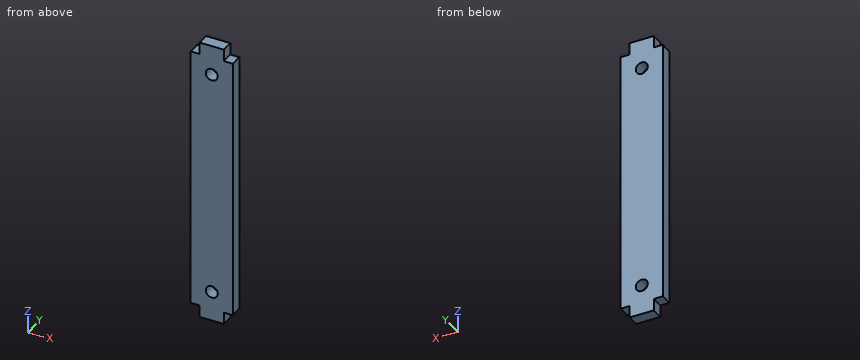
```python
from build123d import *

# Parameters (mm, degrees)
SKETCH1_W           = 17.78
SKETCH1_H           = 111.76
SKETCH1_R           = 2.54
SKETCH1_W_2         = 10.16
SKETCH1_H_2         = 5.08
BOSS_EXTRUDE1_DEPTH = 5.08


with BuildPart() as part:
    # Sketch1 → Boss-Extrude1 (new body)
    with BuildSketch(Plane(origin=(0, 0, 0), x_dir=(1, 0, 0), z_dir=(0, 1, 0))):
        Rectangle(SKETCH1_W, SKETCH1_H)
        with Locations((0, 48.26)):
            Circle(SKETCH1_R, mode=Mode.SUBTRACT)
        with Locations((0, -48.26)):
            Circle(SKETCH1_R, mode=Mode.SUBTRACT)
        with Locations((0, 58.42)):
            Rectangle(SKETCH1_W_2, SKETCH1_H_2)
        with Locations((0, -58.42)):
            Rectangle(SKETCH1_W_2, SKETCH1_H_2)
    extrude(amount=BOSS_EXTRUDE1_DEPTH)


solid = part.part
```
Here's how the part is built. I have some questions about the finished solid (model axes, mm). Give positions to 0.01 mm unless a question says otherwise; leave off trailing zeros. Loops run counter-clockwise (first coordinate to the right, second up) from the corner with the lowest first, then second, coordinate; pieces in that order, holes last. Notation, with made-up numbers: (54.5, 29) -> (60.5, 29) arc R33 cw to (60.5, 65) -> close; hole circle Ø4 at (-9, -25.75). An arc over 180 degrees is marked (long way). Use one line per item in the form item = value. Start each with the question number.
1) Imagine slicing it at B-B (y = 3.15). Please give me the cut outline in (x, z), then the cut area to 3 significant figures.
2) Imagine slicing it at A-A (z = 48.26). Please give me the cut outline in (x, y).
3) For P1, Ø3, axis at x = 7.5, y = 2.5, coming from the +Z side; P2, Ø1.1, axis at x = 6.5, y = 2, coming from the -Z side; P3, Ø2.5, axis at y = 2, z = 58, coming from the -X side, each with a flat end and sliding along its axis, tell me the tip position at first contact or that it passes through.
4) Imagine slicing it at D-D (x = 7.25). Please give me the cut outline in (y, z), then the cut area to 3 significant figures.
5) Please list where these lines run through material, in increasing order: line 1 along Z through (x, y) = (0, 3.65); line 2 along X through (y, z) = (4.45, 50); line 3 along X through (y, z) = (2, -48.26).
6) Imagine slicing it at C-C (x = 0). Please give me the cut outline in (y, z), then the cut area to 3 significant figures.
Check values:
q1.outline = (-8.89, -55.88) -> (-5.08, -55.88) -> (-5.08, -60.96) -> (5.08, -60.96) -> (5.08, -55.88) -> (8.89, -55.88) -> (8.89, 55.88) -> (5.08, 55.88) -> (5.08, 60.96) -> (-5.08, 60.96) -> (-5.08, 55.88) -> (-8.89, 55.88) -> close; hole circle Ø5.08 at (0, -48.26); hole circle Ø5.08 at (0, 48.26)
q1.area = 2,050 mm^2
q2.outline = (-8.89, 0) -> (-2.54, 0) -> (-2.54, 5.08) -> (-8.89, 5.08) -> close; (2.54, 0) -> (8.89, 0) -> (8.89, 5.08) -> (2.54, 5.08) -> close
q3.P1 = 55.88
q3.P2 = -55.88
q3.P3 = -5.08
q4.outline = (0, -55.88) -> (5.08, -55.88) -> (5.08, 55.88) -> (0, 55.88) -> close
q4.area = 568 mm^2
q5.line_1 = -60.96 to -50.8, -45.72 to 45.72, 50.8 to 60.96
q5.line_2 = -8.89 to -1.85, 1.85 to 8.89
q5.line_3 = -8.89 to -2.54, 2.54 to 8.89
q6.outline = (0, -60.96) -> (5.08, -60.96) -> (5.08, -50.8) -> (0, -50.8) -> close; (0, -45.72) -> (5.08, -45.72) -> (5.08, 45.72) -> (0, 45.72) -> close; (0, 50.8) -> (5.08, 50.8) -> (5.08, 60.96) -> (0, 60.96) -> close
q6.area = 568 mm^2
